from build123d import *

# Parameters (mm, degrees)
F0_R     = 16.002
F1_DEPTH = 6.35
F2_W     = 6.35
F2_H     = 76.2
F3_DEPTH = 101.6
F5_DEPTH = 101.6
F6_W     = 6.35
F6_H     = 76.2
F7_DEPTH = 101.6
F9_DEPTH = 25.4


with BuildPart() as f1:
    # F0 (on Top) → F1 (new body)
    with BuildSketch(Plane.XY):
        Polygon((0, -38.1), (0, 0), (-31.75, 0), (-35.56, 0), (-53.34, 0), (-57.15, 0), (-88.9, 0), (-88.9, -76.2), (-57.15, -76.2), (-53.34, -76.2), (-35.56, -76.2), (-31.75, -76.2), (0, -76.2), align=None)
        with Locations((-44.45, -38.1)):
            Circle(F0_R, mode=Mode.SUBTRACT)
        Polygon((-35.56, 0), (-31.75, 0), (-31.75, 2.54), (-31.75, 6.35), (-57.15, 6.35), (-57.15, 2.54), (-57.15, 0), (-53.34, 0), align=None)
        with BuildLine():
            ThreePointArc((-53.34, 1.27), (-54.238026, 1.641974), (-54.61, 2.54))
            ThreePointArc((-54.61, 2.54), (-53.34, 3.81), (-52.07, 2.54))
            ThreePointArc((-52.07, 2.54), (-52.441974, 1.641974), (-53.34, 1.27))
        make_face(mode=Mode.SUBTRACT)
        with BuildLine():
            ThreePointArc((-35.56, 1.27), (-36.458026, 3.438026), (-34.29, 2.54))
            ThreePointArc((-34.29, 2.54), (-34.661974, 1.641974), (-35.56, 1.27))
        make_face(mode=Mode.SUBTRACT)
        Polygon((-31.75, -78.74), (-31.75, -76.2), (-35.56, -76.2), (-53.34, -76.2), (-57.15, -76.2), (-57.15, -78.74), (-57.15, -82.55), (-31.75, -82.55), align=None)
        with BuildLine():
            ThreePointArc((-52.07, -78.74), (-53.34, -80.01), (-54.61, -78.74))
            ThreePointArc((-54.61, -78.74), (-54.238026, -77.841974), (-53.34, -77.47))
            ThreePointArc((-53.34, -77.47), (-52.441974, -77.841974), (-52.07, -78.74))
        make_face(mode=Mode.SUBTRACT)
        with BuildLine():
            ThreePointArc((-35.56, -77.47), (-34.661974, -77.841974), (-34.29, -78.74))
            ThreePointArc((-34.29, -78.74), (-36.458026, -79.638026), (-35.56, -77.47))
        make_face(mode=Mode.SUBTRACT)
    extrude(amount=F1_DEPTH)

    # F2 (on face) → F3 (join)
    with BuildSketch(Plane.XY.offset(6.35)):
        with Locations((-85.725, -38.1)):
            Rectangle(F2_W, F2_H)
    extrude(amount=F3_DEPTH)

    # F4 (on face) → F5 (cut)
    with BuildSketch(Plane(origin=(-88.9, 0, 0), x_dir=(0, -1, 0), z_dir=(-1, 0, 0))):
        with BuildLine():
            ThreePointArc((12.7, 53.975), (38.1, 28.575), (63.5, 53.975))
            ThreePointArc((63.5, 53.975), (38.1, 79.375), (12.7, 53.975))
        make_face()
    extrude(amount=-F5_DEPTH, mode=Mode.SUBTRACT)

    # F6 (on face) → F7 (join)
    with BuildSketch(Plane.XY.offset(6.35)):
        with Locations((-3.175, -38.1)):
            Rectangle(F6_W, F6_H)
    extrude(amount=F7_DEPTH)

    # F8 (on face) → F9 (cut)
    with BuildSketch(Plane.YZ):
        with BuildLine():
            ThreePointArc((-12.7, 53.975), (-20.139488, 71.935512), (-38.1, 79.375))
            ThreePointArc((-38.1, 79.375), (-56.060512, 36.014488), (-12.7, 53.975))
        make_face()
    extrude(amount=-F9_DEPTH, mode=Mode.SUBTRACT)


solid = f1.part
The model under review builds one solid part; all positions refer to its coordinate system, in mm. A direction names the side the tool comes from. Coordinates: 2 decimals unless noted, no trailing zeros. Loops run counter-clockwise (first coordinate to the right, second up) from the corner with the lowest first, then second, coordinate; pieces in that order, holes last. Notation, with made-up numbers: M 40,-8.5 L 57,-8.5 A21 ccw 57,13.5 Z; hole C 36,-24.5 d9. An arc over 180 degrees is marked long. Put each result on its own line as item: value. Start each with the question number.
Q1. Add section B-B (x = -44.45). Write out the cut boundary in (y, z).
Q2. For faces 1 (the flat face through (-6.35, -47, 79)), 2 (the flat face through (-31.75, -79, 3)), 3 (the flat face through (-57.15, -79, 3)), 4 (the flat face through (-5, 0, 42)), list the 3-axis set-ups (+Z, -Z, +X, -X, +Y, -Y) from which the entire face can be reached by the end or side of a thin tool; tool diameter is ignored.
Q3. The part is to be moulded in two halves that separate along Y. For faces 5 (the flat face through (-45, -82.55, 3)), 6 (the flat face through (-31.75, 3, 3)), 7 (the cylindrical face through (-60.437, -37.396, 3.131)), say which applies: +Y half, -Y half, draft (parallel to the pull), parting line (faces both ways), or undercut.
Q4. Wall thickness on line 1 (X direction, y = -78.74, z = 4.5); line 2 (X direction, y = -25.5, z = 91); line 3 (Y direction, x = -44, z = 3): over which ranges is each line inside the solid? List them lowest first.
Q5. Add section A-A (z = 89.5). Write out the cut boundary in (x, y), and give its area (3 significant figures).
Q6. Add section C-C (z = 57). Write out the cut boundary in (x, y), and give its area (3 significant figures).
Q7. Add section D-D (y = -72). Write out the cut boundary in (x, z), and give its area (3 significant figures).
Q8. Clearance check with flat-ended pins moving along their axes: pin 1 (4 mm diameter, centred on x = -9.5, z = 82, fed in from -Y); pin 2 (7 mm diameter, centred on y = -80.5, z = 3, fed in from -X); pin 3 (4 mm diameter, centred on x = -35.56, y = -78.74, fed in from +Z). State where each tip first meets the part, or that it passes through.
Answers:
1. outline: M -82.55,0 L -54.1,0 L -54.1,6.35 L -82.55,6.35 Z; M -22.1,0 L 6.35,0 L 6.35,6.35 L -22.1,6.35 Z
2. face 1: +Z, +Y, -Y
2. face 2: +Z, -Z, +X, -Y
2. face 3: +Z, -Z, -X, -Y
2. face 4: +Z, -Z, +X, +Y
3. face 5: -Y half
3. face 6: draft
3. face 7: undercut
4. line 1: x = -57.15 to -54.61, -52.07 to -36.83, -34.29 to -31.75
4. line 2: x = -88.9 to -82.55, -6.35 to 0
4. line 3: y = -82.55 to -54.1, -22.1 to 6.35
5. outline: M -88.9,-76.2 L -82.55,-76.2 L -82.55,0 L -88.9,0 Z; M -6.35,-76.2 L 0,-76.2 L 0,0 L -6.35,0 Z
5. area: 968 mm^2
6. outline: M -88.9,-76.2 L -82.55,-76.2 L -82.55,-63.32 L -88.9,-63.32 Z; M -88.9,-12.88 L -82.55,-12.88 L -82.55,0 L -88.9,0 Z; M -6.35,-76.2 L 0,-76.2 L 0,-63.32 L -6.35,-63.32 Z; M -6.35,-12.88 L 0,-12.88 L 0,0 L -6.35,0 Z
6. area: 327 mm^2
7. outline: M -88.9,0 L 0,0 L 0,107.95 L -6.35,107.95 L -6.35,6.35 L -82.55,6.35 L -82.55,107.95 L -88.9,107.95 Z
7. area: 1,850 mm^2
8. pin 1: passes through
8. pin 2: stops at x = -57.15
8. pin 3: stops at z = 6.35
